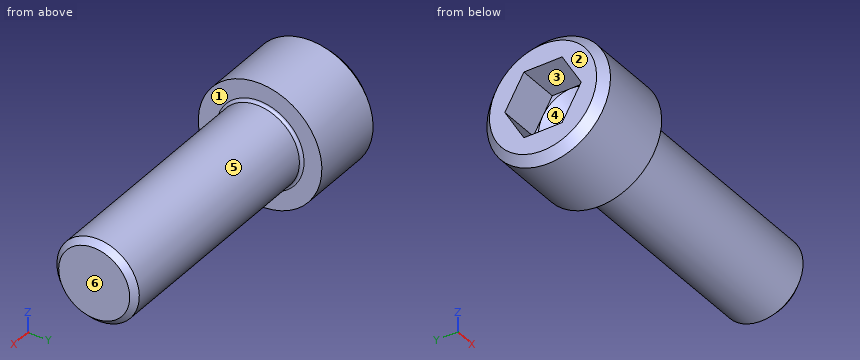
```python
from build123d import *

# Parameters (mm, degrees)
FILLET1_R    = 0.8
HEX_2_DEPTH  = 12
SCALE1_SCALE = 0.1


with BuildPart() as part:
    # BodySke → Base-Revolve (revolve)
    with BuildSketch(Plane.XY, mode=Mode.PRIVATE) as base_revolve_sk:
        Polygon((0, 0), (0, 15.6), (2.4, 18), (24, 18), (24, 12), (92.352, 12), (94, 10.352), (94, 0), align=None)
    revolve(base_revolve_sk.sketch.rotate(Axis((-31.75, 0, 0), (1, 0, 0)), 90), axis=Axis((-31.75, 0, 0), (1, 0, 0)))

    # Fillet1
    fillet1_edges = [part.edges().sort_by_distance(p)[0] for p in [
        (24, 0, -12),
    ]]
    fillet(fillet1_edges, radius=FILLET1_R)

    # Sketch2 → Hex-PreBroach (revolve, cut)
    with BuildSketch(Plane.XY, mode=Mode.PRIVATE) as hex_prebroach_sk:
        Polygon((0, 9.6375), (12, 9.6375), (17.564213219, 0), (0, 0), align=None)
    revolve(hex_prebroach_sk.sketch.rotate(Axis((0, 0, 0), (1, 0, 0)), 90), axis=Axis((0, 0, 0), (1, 0, 0)), mode=Mode.SUBTRACT)

    # Sketch3 → Hex 2 (cut)
    with BuildSketch(Plane(origin=(0, 0, 0), x_dir=(0, 0.500000000000001, 0.866025403784438), z_dir=(-1, 0, 0))):
        Polygon((5.564213219, 9.6375), (-5.564213219, 9.6375), (-11.128426439, 0), (-5.564213219, -9.6375), (5.564213219, -9.6375), (11.128426439, 0), align=None)
    extrude(amount=-HEX_2_DEPTH, mode=Mode.SUBTRACT)


with BuildPart() as part_1:
    # Scale1: scaled about (41.367569692, 0, 0)
    add(part.part.scale(SCALE1_SCALE).moved(Location((37.230812723, 0, 0))))


solid = part_1.part
```
The model under review builds one solid part; all positions refer to its coordinate system, in mm. Face numbers are marked on the shaded views. A direction names the side the tool comes from. Coordinates: 2 decimals unless noted, no trailing zeros. Order: outer loops, then holes, each group sorted by start corner. A loop starts at its lowest first (then second) coordinate and runs counter-clockwise, first axis right, second up. Notation, with made-up numbers: (76, 37.25) -> (131, 37.25) arc R31 cw to (131, 76.25) -> close; hole circle Ø6 at (71, 64.5). An arc over 180 degrees is marked (long way). Answer in a Markdown table with one row per item. Add a question column.
Item 1: Mouldability with a two-part tool opening along Z and no side actions: class the marked faces 4, 5 and 6 as +Z half, -Z half, draft (parallel to the pull), parting line (faces both ways), or undercut.
Item 2: Clearance check with a flat-ended pin moving along its axis: pin 1 (1 mm diameter, centred on y = 0.5, z = 0, fed in from -X). State where the tip first meets the part, or that it passes through.
Item 3: To check wall thickness, follow probe 1 along X at (y, z) = (0.7, 1.2); probe 2 along Y at (x, z) = (38, 0.5); probe 3 along Y at (x, z) = (43, -0.55). State the ranges of each line that lie inside material, in increasing order.
Item 4: Machinability: for the marked faces 1, 2 and 3, which of the approach directions +Z, -Z, +X, -X, +Y, -Y give a long, thin tool a straight path to every point of the face, cutting with its end or side? Answer none if there is none.
Item 5: We need section A-A on x = 43.5. Write out the cut boundary in (y, z), plus the area to 3 significant figures.
Final values:
| question | item | result |
|---|---|---|
| 1 | face 4 | undercut |
| 1 | face 5 | parting line |
| 1 | face 6 | draft |
| 2 | pin 1 | stops at x = 38.43 |
| 3 | probe 1 | x = 37.23 to 39.63 |
| 3 | probe 2 | y = -1.73 to -0.82, 0.82 to 1.73 |
| 3 | probe 3 | y = -1.07 to 1.07 |
| 4 | face 1 | +X |
| 4 | face 2 | +Z, -Z, -X, +Y, -Y |
| 4 | face 3 | -X |
| 5 | outline | circle Ø2.4 at (0, 0) |
| 5 | area | 4.52 mm2 |
